Geometry check sheet. Reference: the model listing, model coordinates, mm. A direction names the side the tool comes from. Give positions to 0.01 mm unless a question says otherwise; leave off trailing zeros. Write each loop counter-clockwise with the first axis right and the second up, starting at its lowest first coordinate (ties: lowest second). Pieces come first, ordered by that corner, then holes. Notation, with made-up numbers: (-32, -29) - (22, -29) arc R7 ccw to (22, -22) - close; hole circle Ø4 at (89, 2.25). An arc over 180 degrees is marked (long way). Use a Markdown table: item, result.
```python
from build123d import *

# Parameters (mm, degrees)
F1_DEPTH = 57.15
F2_R     = 3.175
F3_R     = 28.57499
F5_D     = 25.4
F5_DEPTH = 38.1
F5_TIP   = 7.6309298617
F6_D     = 25.4
F7_R     = 38.1
F9_DEPTH = 15.875


# Not quite as in the source:
# - a fillet or chamfer is up to 0.001 mm smaller than in the source, because OpenCascade refuses the exact size
# - a length typed as a fraction of an inch, garbled in the dataset ("3 / 203.2 mm" for 3/8 in), is restored


with BuildPart() as f1:
    # F0 (on Top) → F1 (new body)
    with BuildSketch(Plane.XY):
        with BuildLine():
            ThreePointArc((28.575, -6.35), (30.4348719395, -1.8598719395), (34.925, 0))
            Line((34.925, 0), (228.6, 0))
            Line((228.6, 0), (228.6, 15.875))
            Line((228.6, 15.875), (34.925, 15.875))
            ThreePointArc((34.925, 15.875), (30.4348719395, 17.7348719395), (28.575, 22.225))
            Line((28.575, 22.225), (28.575, 36.5125))
            Line((28.575, 36.5125), (0, 36.5125))
            Line((0, 36.5125), (-28.575, 36.5125))
            Line((-28.575, 36.5125), (-28.575, 22.225))
            ThreePointArc((-28.575, 22.225), (-30.4348719395, 17.7348719395), (-34.925, 15.875))
            Line((-34.925, 15.875), (-304.8, 15.875))
            Line((-304.8, 15.875), (-304.8, 0))
            Line((-304.8, 0), (-34.925, 0))
            ThreePointArc((-34.925, 0), (-30.4348719395, -1.8598719395), (-28.575, -6.35))
            Line((-28.575, -6.35), (-28.575, -20.6375))
            Line((-28.575, -20.6375), (0, -20.6375))
            Line((0, -20.6375), (28.575, -20.6375))
            Line((28.575, -20.6375), (28.575, -6.35))
        make_face()
    extrude(amount=F1_DEPTH)

    # F2
    f2_edges = [f1.edges().sort_by_distance(p)[0] for p in [
        (28.575, 36.5125, 28.575),
        (0, 36.5125, 57.15),
        (-28.575, 36.5125, 28.575),
        (0, 36.5125, 0),
        (-28.575, -20.6375, 28.575),
        (0, -20.6375, 57.15),
        (28.575, -20.6375, 28.575),
        (0, -20.6375, 0),
    ]]
    fillet(f2_edges, radius=F2_R)

    # F3 (radius 28.575 in the source; OpenCascade refuses exactly that, so slightly less here)
    f3_edges = [f1.edges().sort_by_distance(p)[0] for p in [
        (-304.8, 7.9375, 57.15),
        (-304.8, 7.9375, 0),
    ]]
    fillet(f3_edges, radius=F3_R)

    # F5 (one way)
    with BuildSketch(Plane.XZ):
        with Locations((0, 28.575)):
            Circle(F5_D / 2)
    extrude(amount=-F5_DEPTH, mode=Mode.SUBTRACT)
    with Locations(Plane.XZ):
        with Locations((0, 28.575)):
            with Locations((0, 0, -(F5_DEPTH + F5_TIP / 2))):  # 118° drill point
                Cone(0, F5_D / 2, F5_TIP, mode=Mode.SUBTRACT)

    # F6 (through all)
    with Locations(Plane(origin=(0, 0, 0), x_dir=(1, 0, 0), z_dir=(0, 1, 0))):
        with Locations((0, -28.575)):
            Hole(F6_D / 2)

    # F7
    f7_edges = [f1.edges().sort_by_distance(p)[0] for p in [
        (228.6, 7.9375, 57.15),
    ]]
    fillet(f7_edges, radius=F7_R)

    # F8 (on Top) → F9 (join)
    with BuildSketch(Plane.XY):
        Polygon((228.6, -76.2), (228.6, 0), (228.6, 92.075), (171.45, 92.075), (171.45, -76.2), align=None)
    extrude(amount=-F9_DEPTH)


solid = f1.part
```
1) Depth check by flat-ended pin: P1, Ø5, axis at x = -188, z = -4.5, coming from the -Y side; P2, Ø3.5, axis at y = 29, z = 25.5, coming from the +X side (3 decimals); P3, Ø10, axis at y = -1.5, z = 16, coming from the +X side; P4, Ø6, axis at y = -1.5, z = 25, coming from the -X side. Enter the tip coordinate at first touch or a pass-through.
Working result:
| item | result |
|---|---|
| P1 | passes through |
| P2 | stops at x = 28.575 |
| P3 | stops at x = 228.6 |
| P4 | stops at x = -304.78 |
2) Set-up check for faces 1 (the flat face through (133, 15.875, 28)), 2 (the flat face through (28.575, -12, 28)), 3 (the flat face through (-56, 8, 0)), 4 (the flat face through (-28.575, 28, 28)), 5 (the flat face through (-28.575, -12, 28)): record each of +Z, -Z, +X, -X, +Y, -Y from which the full face is reachable in a straight line by a thin tool's end or side.
Working result:
| item | result |
|---|---|
| face 1 | +Z, +X, +Y |
| face 2 | +Z, -Z, +X, -Y |
| face 3 | -Z, -X, +Y, -Y |
| face 4 | +Z, -Z, -X, +Y |
| face 5 | +Z, -Z, -X, -Y |
3) Material ranges on L1, parallel to Z at x = 0, y = -14.25 (3 decimals); L2, parallel to X at y = -14.5, z = 50 (3 decimals); L3, parallel to Y at x = 90, z = 37 (3 decimals), recorded low to high. Write a range as from..to.
Working result:
| item | result |
|---|---|
| L1 | z = 0..15.875, 41.275..57.15 |
| L2 | x = -28.575..28.575 |
| L3 | y = 0..15.875 |
4) Section check D-D on x = -242. Record the boundary of the cut face in (y, z) (3 decimals), then the cut area to 3 significant figures.
Working result:
| item | result |
|---|---|
| outline | (0, 0) - (15.875, 0) - (15.875, 57.15) - (0, 57.15) - close |
| area | 907 mm² |
5) Section check C-C on y = 67. Record the boundary of the cut face in (x, z) (3 decimals).
Working result:
| item | result |
|---|---|
| outline | (171.45, -15.875) - (228.6, -15.875) - (228.6, 0) - (171.45, 0) - close |
